from build123d import *

# Parameters (mm, degrees)
ESQUISSE2_R                  = 1
ESQUISSE2_R_2                = 0.25
ENL_V_MAT_EXTRU_1_DEPTH      = 10
R_P_TITION_CIRCULAIRE1_COUNT = 2


with BuildPart() as part:
    # Esquisse1 → Révolution1 (revolve)
    with BuildSketch(Plane.XY, mode=Mode.PRIVATE) as r_volution1_sk:
        Polygon((4, 0), (4, 5), (1.5, 5), (1.5, 6.5), (3.5, 6.5), (3.5, 8.5), (4.5, 8.5), (4.5, 8), (19.8, 8), (19.8, 3), (6, 3), (6, 0), align=None)
    revolve(r_volution1_sk.sketch.rotate(Axis((0, 0, 0), (0, 1, 0)), 90), axis=Axis((0, 0, 0), (0, 1, 0)))

    # Esquisse2 → Enlèv. mat.-Extru.1 (cut)
    with BuildSketch(Plane(origin=(0, 8, 0), x_dir=(1, 0, 0), z_dir=(0, 1, 0))):
        with Locations(Location((0, 16.5, 0), (0, 0, 270))):
            Circle(ESQUISSE2_R)
        with Locations(Location((0, 11.5, 0), (0, 0, 270))):
            Circle(ESQUISSE2_R)
        with Locations(Location((0, 5, 0), (0, 0, 270))):
            Circle(ESQUISSE2_R_2)
        with Locations(Location((7.424621202, 7.424621202, 0), (0, 0, 270))):
            Circle(ESQUISSE2_R)
        with Locations(Location((10.960155108, 10.960155108, 0), (0, 0, 270))):
            Circle(ESQUISSE2_R)
        with Locations(Location((11, 0, 0), (0, 0, 270))):
            Circle(ESQUISSE2_R)
        with Locations(Location((16, 0, 0), (0, 0, 270))):
            Circle(ESQUISSE2_R)
        with Locations(Location((10.606601718, -10.606601718, 0), (0, 0, 270))):
            Circle(ESQUISSE2_R)
        with Locations(Location((7.071067812, -7.071067812, 0), (0, 0, 270))):
            Circle(ESQUISSE2_R)
    enl_v_mat_extru_1 = extrude(amount=-ENL_V_MAT_EXTRU_1_DEPTH, mode=Mode.SUBTRACT)

    # Répétition circulaire1: Enlèv. mat.-Extru.1 ×2 about axis
    r_p_tition_circulaire1_axis = Axis((0, 0, 0), (0, 1, 0))
    for i in range(1, R_P_TITION_CIRCULAIRE1_COUNT):
        add(enl_v_mat_extru_1.rotate(r_p_tition_circulaire1_axis, i * 360 / R_P_TITION_CIRCULAIRE1_COUNT), mode=Mode.SUBTRACT)


solid = part.part
Geometry: final body of the model. Coordinates: model frame, mm. A direction names the side the tool comes from. Coordinates: 2 decimals unless noted, no trailing zeros. Loops run counter-clockwise (first coordinate to the right, second up) from the corner with the lowest first, then second, coordinate; pieces in that order, holes last. Notation, with made-up numbers: (81.5, 3) - (85.5, 3) arc R17 ccw to (85.5, 17) - close; hole circle Ø9 at (-16, 36.25). An arc over 180 degrees is marked (long way). One line per question, with ' | ' between items. Start each with the question number.
(1) Cut plane B-B on x = 16. Output: boundary loops of the cut face in (y, z), and give its area (3 significant figures).
(2) Ray query, L1, parallel to X at y = 6.05, z = -11.5; L2, parallel to X at y = 7, z = -7.5; L3, parallel to Z at x = -0.5, y = 6. Return the intervals inside material, ascending. Write a range as from..to.
(3) First-contact query: pin 1 (3 mm diameter, centred on x = -10.96, z = 10.96, fed in from -Y); pin 2 (2 mm diameter, centred on x = 14.5, y = 2.5, fed in from -Z); pin 3 (8 mm diameter, centred on x = -10, z = -13.5, fed in from +Y); pin 4 (9 mm diameter, centred on x = 0, z = 0, fed in from +Y). Flat tips, straight axial feed; report the tip coordinate or a pass-through.
(4) Cut plane C-C on y = 6. Count the separate pieces of the cut face and the enclosed holes in it, and give its area (3 significant figures).
(5) Draft query along Z for faces 1 (the flat face through (4, 3, 5)), 2 (the flat face through (2, 6.5, 0)), 3 (the cylindrical face through (-10, 6, 0)), 4 (the cylindrical face through (-5.9, 5.5, -18.9)). Return one class per face: +Z half, -Z half, draft (parallel to the pull), parting line (faces both ways), or undercut.
(6) Cut plane A-A on z = 16.5. Output: boundary loops of the cut face in (x, y).
(7) Cut plane D-D on z = 7. Output: boundary loops of the cut face in (x, y).
(8) Reachability of faces 5 (the flat face through (0, 5, -2)), 6 (the cylindrical face through (3.105, 7.514, -1.615)), 7 (the cylindrical face through (-15, 6, 0)) from +Z, -Z, +X, -X, +Y, -Y: full face, straight path, thin tool, end or side. Return the list, or none.
Here are the results:
1) outline: (3, -11.66) - (8, -11.66) - (8, -1) - (3, -1) - close; (3, 1) - (8, 1) - (8, 11.66) - (3, 11.66) - close | area: 107 mm²
2) L1: -16.12..-11.06, -10.16..-1, 1..10.12, 11.8..16.12 | L2: -18.32..-7.97, -6.17..6.43, 8.42..18.32 | L3: -19.79..-17.37, -15.63..-12.37, -10.63..-1.41, 1.41..10.63, 12.37..15.63, 17.37..19.79
3) pin 1: y = 3 | pin 2: z = -14.36 | pin 3: y = 8 | pin 4: y = 8.5
4) separate pieces: 1 | enclosed holes: 19 | area: 1,170 mm²
5) face 1: draft | face 2: undercut | face 3: undercut | face 4: parting line
6) outline: (-10.94, 3) - (-1, 3) - (-1, 8) - (-10.94, 8) - close; (1, 3) - (10.94, 3) - (10.94, 8) - (1, 8) - close
7) outline: (-18.52, 3) - (-8.33, 3) - (-8.33, 8) - (-18.52, 8) - close; (-6.52, 3) - (6.07, 3) - (6.07, 8) - (-6.52, 8) - close; (8.07, 3) - (18.52, 3) - (18.52, 8) - (8.07, 8) - close
8) face 5: -Y | face 6: +Y | face 7: +Y, -Y
